from build123d import *

# Parameters (mm, degrees)
SKETCH_1_W      = 45
SKETCH_1_H      = 40
SKETCH_1_R      = 2.5
EXTRUDE_1_DEPTH = 3
EXTRUDE_START   = 22.5
SKETCH_2_W      = 7
SKETCH_2_H      = 40
EXTRUDE_2_DEPTH = 3


with BuildPart() as part:
    # 草圖1 → 填料-伸長1 (new body)
    with BuildSketch(Plane.XY):
        Rectangle(SKETCH_1_W, SKETCH_1_H)
        with Locations((-12.5, 0)):
            Circle(SKETCH_1_R, mode=Mode.SUBTRACT)
    extrude(amount=EXTRUDE_1_DEPTH)

    # 草圖2 → 填料-伸長2 (add)
    with BuildSketch(Plane(origin=(0, 0, 0), x_dir=(0, 0, -1), z_dir=(1, 0, 0)).offset(EXTRUDE_START)):
        with Locations((-1.5, 0)):
            Rectangle(SKETCH_2_W, SKETCH_2_H)
    extrude(amount=EXTRUDE_2_DEPTH)


solid = part.part
Design review of the part built by this model. Coordinates are the model's own, in mm. A direction names the side the tool comes from. Round coordinates to 2 decimals unless told otherwise and drop trailing zeros. Write each loop counter-clockwise with the first axis right and the second up, starting at its lowest first coordinate (ties: lowest second). Pieces come first, ordered by that corner, then holes.
Item 1: Consider section C-C on y = 13. Give the boundary of the cut face in (x, z), and give its area (3 significant figures).
Item 2: Consider section D-D on z = 4. Give the boundary of the cut face in (x, y).
Item 3: Draft analysis for pull direction X (two halves, no side actions). For faces 1 (the flat face through (22.5, 0, -1)), 2 (the cylindrical face through (-15, 0, 1)), 3 (the flat face through (0, 0, 0)), 4 (the flat face through (25.5, 0, 2)), state which applies: released by +X, released by -X, zero draft, split by the parting line, or undercut.
Item 4: For pin 1 Ø12 at (x, y) = (-9, 8.5) entering from -Z; pin 2 Ø1.5 at (x, y) = (-14, -8) entering from +Z; pin 3 Ø2 at (y, z) = (-5.5, 3.5) entering from -X; pin 4 Ø1 at (y, z) = (-4.5, -1) entering from -X, all flat-tipped, find the tip position at first contact; note any pin that passes through.
Item 5: Consider section A-A on x = -12.5. Give the boundary of the cut face in (y, z), and give its area (3 significant figures).
Item 6: Consider section B-B on y = 0. Give the boundary of the cut face in (x, z).
Item 7: Wall thickness on L1, parallel to Y at x = -12.5, z = 1; L2, parallel to Z at x = -8.5, y = -17.5; L3, parallel to X at y = -1.5, z = 0.25: over which ranges is each line inside the solid? List them lowest first.
Item 8: For faces 5 (the flat face through (0, 0, 3)), 6 (the flat face through (5, 20, 2)), list the 3-axis set-ups (+Z, -Z, +X, -X, +Y, -Y) from which the entire face can be reached by the end or side of a thin tool; tool diameter is ignored.
Check values:
1. outline: (-22.5, 0) - (22.5, 0) - (22.5, -2) - (25.5, -2) - (25.5, 5) - (22.5, 5) - (22.5, 3) - (-22.5, 3) - close
1. area: 156 mm2
2. outline: (22.5, -20) - (25.5, -20) - (25.5, 20) - (22.5, 20) - close
3. face 1: released by -X
3. face 2: undercut
3. face 3: zero draft
3. face 4: released by +X
4. pin 1: stops at z = 0
4. pin 2: stops at z = 3
4. pin 3: stops at x = -22.5
4. pin 4: stops at x = 22.5
5. outline: (-20, 0) - (-2.5, 0) - (-2.5, 3) - (-20, 3) - close; (2.5, 0) - (20, 0) - (20, 3) - (2.5, 3) - close
5. area: 105 mm2
6. outline: (-22.5, 0) - (-15, 0) - (-15, 3) - (-22.5, 3) - close; (-10, 0) - (22.5, 0) - (22.5, -2) - (25.5, -2) - (25.5, 5) - (22.5, 5) - (22.5, 3) - (-10, 3) - close
7. L1: y = -20 to -2.5, 2.5 to 20
7. L2: z = 0 to 3
7. L3: x = -22.5 to -14.5, -10.5 to 25.5
8. face 5: +Z, -X, +Y, -Y
8. face 6: +Z, -Z, +X, -X, +Y
